from build123d import *

# Parameters (mm, degrees)
BOSS_EXTRUDE1_DEPTH = 1.5875
FILLET1_R           = 2
FILLET3_R           = 8
FILLET4_R           = 8


with BuildPart() as part:
    # Sketch3 → Boss-Extrude1 (new body)
    with BuildSketch(Plane.XY):
        Polygon((58.775, 33.228336454), (53.202823644, 29.668334894), (46.775, 25.561669788), (40.347176356, 29.668334894), (34.775, 33.228336454), (22.775, 25.561669788), (14.005335663, 31.164510892), (7.544664337, 21.052155774), (22.775, 11.321663546), (28.347176356, 14.881665106), (34.775, 18.988330212), (41.202823644, 14.881665106), (46.775, 11.321663546), (58.775, 18.988330212), (67.544664337, 13.385489108), (74.005335663, 23.497844226), align=None)
    extrude(amount=BOSS_EXTRUDE1_DEPTH)

    # Fillet1
    fillet1_edges = [part.edges().sort_by_distance(p)[0] for p in [
        (7.544664337, 21.052155774, 0.79375),
        (14.005335663, 31.164510892, 0.79375),
        (74.005335663, 23.497844226, 0.79375),
        (67.544664337, 13.385489108, 0.79375),
    ]]
    fillet(fillet1_edges, radius=FILLET1_R)

    # Fillet3
    fillet3_edges = [part.edges().sort_by_distance(p)[0] for p in [
        (46.775, 11.321663546, 0.79375),
        (22.775, 11.321663546, 0.79375),
        (34.775, 33.228336454, 0.79375),
        (58.775, 33.228336454, 0.79375),
    ]]
    fillet(fillet3_edges, radius=FILLET3_R)

    # Fillet4
    fillet4_edges = [part.edges().sort_by_distance(p)[0] for p in [
        (34.775, 18.988330212, 0.79375),
        (22.775, 25.561669788, 0.79375),
        (46.775, 25.561669788, 0.79375),
        (58.775, 18.988330212, 0.79375),
    ]]
    fillet(fillet4_edges, radius=FILLET4_R)


solid = part.part
Design review of the part built by this model. Coordinates are the model's own, in mm. A direction names the side the tool comes from. Round coordinates to 2 decimals unless told otherwise and drop trailing zeros. Order: outer loops, then holes, each group sorted by start corner. A loop starts at its lowest first (then second) coordinate and runs counter-clockwise, first axis right, second up.
1) Machinability: for faces 1 (the cylindrical face through (8.35, 21.25, 0.8)), 2 (the flat face through (52.75, 15.14, 0.78)), 3 (the flat face through (28.8, 29.41, 0.78)), which of the approach directions +Z, -Z, +X, -X, +Y, -Y give a long, thin tool a straight path to every point of the face, cutting with its end or side? Answer none if there is none.
The answers:
face 1: +Z, -Z, -X
face 2: +Z, -Z, -Y
face 3: +Z, -Z, +Y
2) Consider section B-B (y = 18.75). State the section outline as (x, z) points, plus the area to 3 significant figures.
The answers:
outline: (11.15, 0) - (70.97, 0) - (70.97, 1.59) - (11.15, 1.59) - close
area: 95.0 mm2
3) Consider section A-A (z = 0.95). State the section outline as (x, y) points (3 decimals).
The answers:
outline: (8.621, 22.738) arc R2 ccw to (9.23, 19.975) - (18.468, 14.073) arc R8 ccw to (27.082, 14.073) - (30.468, 16.237) arc R8 cw to (39.082, 16.237) - (42.468, 14.073) arc R8 ccw to (51.082, 14.073) - (54.468, 16.237) arc R8 cw to (63.082, 16.237) - (65.859, 14.462) arc R2 ccw to (68.621, 15.071) - (72.929, 21.812) arc R2 ccw to (72.32, 24.575) - (63.082, 30.477) arc R8 ccw to (54.468, 30.477) - (51.082, 28.313) arc R8 cw to (42.468, 28.313) - (39.082, 30.477) arc R8 ccw to (30.468, 30.477) - (27.082, 28.313) arc R8 cw to (18.468, 28.313) - (15.691, 30.088) arc R2 ccw to (12.929, 29.479) - close
4) For L1, parallel to X at y = 14.5, z = 0.8; L2, parallel to X at y = 29.75, z = 1.2; L3, parallel to Y at x = 47, z = 0.55, list the stretches that pass through material, from the lowest coordinate up.
The answers:
L1: x = 17.8 to 27.75, 41.8 to 51.75, 65.8 to 68.07
L2: x = 13.14 to 16.22, 29.33 to 40.22, 53.33 to 64.22
L3: y = 12.82 to 27.06
5) Consider section C-C (x = 47). State the section outline as (y, z) points, plus the area to 3 significant figures.
The answers:
outline: (12.82, 0) - (27.06, 0) - (27.06, 1.59) - (12.82, 1.59) - close
area: 22.6 mm2
6) Clearance check with a flat-ended pin moving along its axis: pin 1 Ø3 at (x, y) = (35.5, 15.5) entering from -Z. State where the tip first meets the part, or that it passes through.
The answers:
pin 1: passes through
7) Draft analysis for pull direction X (two halves, no side actions). For faces 4 (the flat face through (40, 22, 0)), 5 (the cylindrical face through (22.839, 27.055, 0.805)), 6 (the flat face through (10.81, 26.16, 0.78)), state which applies: released by +X, released by -X, zero draft, split by the parting line, or undercut.
The answers:
face 4: zero draft
face 5: undercut
face 6: released by -X
